```python
from build123d import *

# Parameters (mm, degrees)
SKETCH1_W                    = 1430
SKETCH1_H                    = 72
BASE_FLANGE1_DEPTH           = 1.5
EDGE_FLANGE1_STRIP_W         = 7.4732
EDGE_FLANGE1_STRIP_H         = 1.5
EDGE_FLANGE1_STRIP_CUT_DEPTH = 1430
EDGE_FLANGE1_DEPTH           = 1430
EDGE_FLANGE2_STRIP_W         = 7.4732
EDGE_FLANGE2_STRIP_H         = 1.5
EDGE_FLANGE2_STRIP_CUT_DEPTH = 1430
EDGE_FLANGE2_DEPTH           = 1430
CUT_EXTRUDE1_START           = -912.816666667
CUT_EXTRUDE1_DEPTH           = 30
CUT_EXTRUDE2_START           = 487.183333333
CUT_EXTRUDE2_DEPTH           = 30
SKETCH14_R                   = 3.25
CUT_EXTRUDE3_DEPTH           = 10


# Read off the part's stored shape, not the designer's step: Cut-Extrude1, Cut-Extrude2
# Sheet-metal steps are written as plain solids
with BuildPart() as part:
    # Sketch1 → Base-Flange1 (new body)
    with BuildSketch(Plane.XY):
        with Locations((-197.816666667, 186.841666667)):
            Rectangle(SKETCH1_W, SKETCH1_H)
    extrude(amount=-BASE_FLANGE1_DEPTH)

    # Edge-Flange1 strip (across the edge) → Edge-Flange1 strip cut (cut)
    with BuildSketch(Plane(origin=(517.183333333, 222.841666667, 0), x_dir=(0, -1, 0), z_dir=(-1, 0, 0))):
        with Locations((-1.5, -0.75)):
            Rectangle(EDGE_FLANGE1_STRIP_W, EDGE_FLANGE1_STRIP_H)
    extrude(amount=EDGE_FLANGE1_STRIP_CUT_DEPTH, mode=Mode.SUBTRACT)

    # Edge-Flange1 section (across the edge) → Edge-Flange1 (add)
    with BuildSketch(Plane(origin=(517.183333333, 222.841666667, 0), x_dir=(0, -1, 0), z_dir=(-1, 0, 0))):
        with BuildLine():
            Line((0, 0.7366), (0, 13.5))
            Line((0, 13.5), (1.5, 13.5))
            Line((1.5, 13.5), (1.5, 0.7366))
            ThreePointArc((1.5, 0.7366), (1.715745145, 0.215745145), (2.2366, 0))
            Line((2.2366, 0), (2.2366, -1.5))
            ThreePointArc((2.2366, -1.5), (0.655084973, -0.844915027), (0, 0.7366))
        make_face()
    extrude(amount=EDGE_FLANGE1_DEPTH)

    # Edge-Flange2 strip (across the edge) → Edge-Flange2 strip cut (cut)
    with BuildSketch(Plane(origin=(-912.816666667, 150.841666667, 0), x_dir=(0, 1, 0), z_dir=(1, 0, 0))):
        with Locations((-1.5, -0.75)):
            Rectangle(EDGE_FLANGE2_STRIP_W, EDGE_FLANGE2_STRIP_H)
    extrude(amount=EDGE_FLANGE2_STRIP_CUT_DEPTH, mode=Mode.SUBTRACT)

    # Edge-Flange2 section (across the edge) → Edge-Flange2 (add)
    with BuildSketch(Plane(origin=(-912.816666667, 150.841666667, 0), x_dir=(0, 1, 0), z_dir=(1, 0, 0))):
        with BuildLine():
            Line((0, 0.7366), (0, 13.5))
            Line((0, 13.5), (1.5, 13.5))
            Line((1.5, 13.5), (1.5, 0.7366))
            ThreePointArc((1.5, 0.7366), (1.715745145, 0.215745145), (2.2366, 0))
            Line((2.2366, 0), (2.2366, -1.5))
            ThreePointArc((2.2366, -1.5), (0.655084973, -0.844915027), (0, 0.7366))
        make_face()
    extrude(amount=EDGE_FLANGE2_DEPTH)

    # Cut-Extrude1 outline → Cut-Extrude1 (cut)
    with BuildSketch(Plane.YZ.offset(CUT_EXTRUDE1_START)):
        with BuildLine():
            ThreePointArc((150.841666667, 0.7366), (151.49675164, -0.844915027), (153.078266667, -1.5))
            Line((153.078266667, -1.5), (153.078266667, 0))
            ThreePointArc((153.078266667, 0), (152.557411812, 0.215745145), (152.341666667, 0.7366))
            Line((152.341666667, 0.7366), (152.341666667, 13.5))
            Line((152.341666667, 13.5), (150.841666667, 13.5))
            Line((150.841666667, 13.5), (150.841666667, 0.7366))
        make_face()
        with BuildLine():
            ThreePointArc((221.341666667, 0.7366), (221.125921522, 0.215745145), (220.605066667, 0))
            Line((220.605066667, 0), (220.605066667, -1.5))
            ThreePointArc((220.605066667, -1.5), (222.186581693, -0.844915026), (222.841666667, 0.7366))
            Line((222.841666667, 0.7366), (222.841666667, 13.5))
            Line((222.841666667, 13.5), (221.341666667, 13.5))
            Line((221.341666667, 13.5), (221.341666667, 0.7366))
        make_face()
    extrude(amount=CUT_EXTRUDE1_DEPTH, mode=Mode.SUBTRACT)

    # Cut-Extrude2 outline → Cut-Extrude2 (cut)
    with BuildSketch(Plane.YZ.offset(CUT_EXTRUDE2_START)):
        with BuildLine():
            ThreePointArc((150.841666667, 0.7366), (151.49675164, -0.844915027), (153.078266667, -1.5))
            Line((153.078266667, -1.5), (153.078266667, 0))
            ThreePointArc((153.078266667, 0), (152.557411812, 0.215745145), (152.341666667, 0.7366))
            Line((152.341666667, 0.7366), (152.341666667, 13.5))
            Line((152.341666667, 13.5), (150.841666667, 13.5))
            Line((150.841666667, 13.5), (150.841666667, 0.7366))
        make_face()
        with BuildLine():
            ThreePointArc((221.341666667, 0.7366), (221.125921522, 0.215745145), (220.605066667, 0))
            Line((220.605066667, 0), (220.605066667, -1.5))
            ThreePointArc((220.605066667, -1.5), (222.186581693, -0.844915026), (222.841666667, 0.7366))
            Line((222.841666667, 0.7366), (222.841666667, 13.5))
            Line((222.841666667, 13.5), (221.341666667, 13.5))
            Line((221.341666667, 13.5), (221.341666667, 0.7366))
        make_face()
    extrude(amount=CUT_EXTRUDE2_DEPTH, mode=Mode.SUBTRACT)

    # Sketch14 → Cut-Extrude3 (cut)
    with BuildSketch(Plane.XY):
        with Locations((502.183333333, 186.841666667)):
            Circle(SKETCH14_R)
        with Locations((-897.816666667, 186.841666667)):
            Circle(SKETCH14_R)
    extrude(amount=-CUT_EXTRUDE3_DEPTH, mode=Mode.SUBTRACT)


solid = part.part
```
Verification items for the finished model (mm, model axes). Coordinates: 2 decimals unless noted, no trailing zeros. Loops run counter-clockwise (first coordinate to the right, second up) from the corner with the lowest first, then second, coordinate; pieces in that order, holes last. Notation, with made-up numbers: (39.5, 73) - (50.5, 73) arc R13 ccw to (50.5, 80) - close; hole circle Ø11 at (29, 47). An arc over 180 degrees is marked (long way). Answer as a JSON object with one key per item and string values.
(1) Cross-section at A-A, the plane z = 7.75. Record the boundary of the cut face in (x, y), then the cut area to 3 significant figures.
Response:
{"outline": "(-882.82, 150.84) - (487.18, 150.84) - (487.18, 152.34) - (-882.82, 152.34) - close; (-882.82, 221.34) - (487.18, 221.34) - (487.18, 222.84) - (-882.82, 222.84) - close", "area": "4,110 mm²"}
(2) Mould release check, pull along Y, two halves, no side actions. Record for faces 1 (the flat face through (-208, 187, -1.5)), 2 (the flat face through (-208, 187, 0)): pulls with the +Y half, pulls with the -Y half, needs draft (parallel to the pull), parting line crosses it, or undercut.
Response:
{"face 1": "needs draft", "face 2": "undercut"}
(3) Cross-section at C-C, the plane y = 172.5. Record the boundary of the cut face in (x, z).
Response:
{"outline": "(-912.82, -1.5) - (517.18, -1.5) - (517.18, 0) - (-912.82, 0) - close"}
(4) Cross-section at B-B, the plane x = 354. Record the boundary of the cut face in (y, z).
Response:
{"outline": "(150.84, 0.74) arc R2.24 ccw to (153.08, -1.5) - (220.61, -1.5) arc R2.24 ccw to (222.84, 0.74) - (222.84, 13.5) - (221.34, 13.5) - (221.34, 0.74) arc R0.74 cw to (220.61, 0) - (153.08, 0) arc R0.74 cw to (152.34, 0.74) - (152.34, 13.5) - (150.84, 13.5) - close"}
(5) Go/stop test with flat-tipped pins: pin 1 Ø1.8 at (y, z) = (222, 4) entering from +X; pin 2 Ø0.7 at (y, z) = (152, 6.5) entering from -X; pin 3 Ø7.5 at (x, y) = (-897.82, 186.84) entering from +Z. Record where each tip stops, or that it passes through.
Response:
{"pin 1": "stops at x = 487.18", "pin 2": "stops at x = -882.82", "pin 3": "stops at z = 0"}
(6) Scan lines: line 1 along Y through (x, z) = (-673.5, 4); line 2 along Y through (x, z) = (408, 0.5); line 3 along Z through (x, y) = (-570, 174.5). Record each from-to range of solid material in increasing order.
Response:
{"line 1": "y = 150.84 to 152.34, 221.34 to 222.84", "line 2": "y = 150.85 to 152.38, 221.3 to 222.83", "line 3": "z = -1.5 to 0"}
